Source: CAD feature listing. Evaluate the final solid. Frame: model axes, mm. Face numbers are marked on the shaded views. A direction names the side the tool comes from. Give positions to 0.01 mm unless a question says otherwise; leave off trailing zeros.
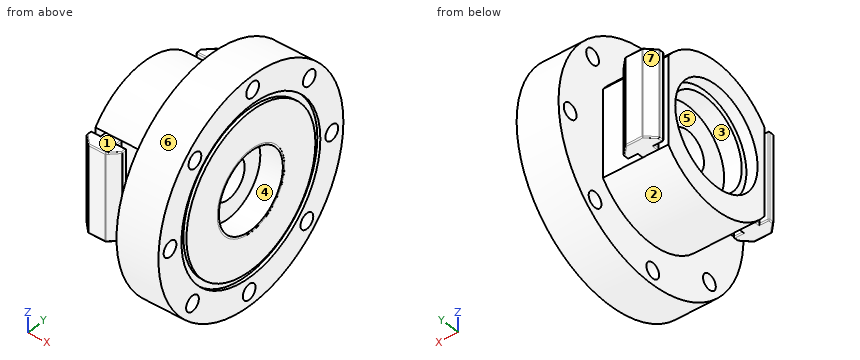
```python
from build123d import *

# Parameters (mm, degrees)
M6_CLEARANCE_HOLE1_D = 7
SKETCH4_W            = 29.717000002
SKETCH4_H            = 66.04
CUT_EXTRUDE1_DEPTH   = 6.5786
BOSS_EXTRUDE1_DEPTH  = 39.556176
FILLET1_R            = 0.508
FILLET1_OF_MIRROR1_R = 0.508


with BuildPart() as part:
    # Main sketch → Revolve1 (revolve)
    with BuildSketch(Plane.XY):
        Polygon((0, 9.000000034), (0, 20.074999982), (-8.000000002, 20.074999982), (-8.000000002, 22.614999982), (-13.080000002, 22.614999982), (-13.080000002, 33.02), (-8.000000002, 33.02), (16.637, 33.02), (16.637, 50.8), (35.687, 50.8), (35.687, 38.1508), (34.3154, 38.1508), (34.3154, 35.433), (35.687, 35.433), (35.687, 18.4912), (35.6616, 18.4912), (35.6616, 17.6022), (25.4, 17.6022), (25.4, 9.000000034), align=None)
    revolve(axis=Axis((71.950113838, 0, 0), (-1, 0, 0)))

    # M6 Clearance Hole1 (through all)
    with Locations(Plane(origin=(35.687, 0, 0), x_dir=(0, 0, -1), z_dir=(1, 0, 0))):
        with Locations((0, 0), (-44.439876155, 0.948634466), (-32.094523648, -30.75295192), (-0.948634466, -44.439876155), (30.75295192, -32.094523648), (44.439876155, -0.948634466), (32.094523648, 30.75295192), (0.948634466, 44.439876155), (-30.75295192, 32.094523648)):
            Hole(M6_CLEARANCE_HOLE1_D / 2)

    # Sketch4 → Cut-Extrude1 (cut)
    with BuildSketch(Plane(origin=(0, 33.02, 0), x_dir=(1, 0, 0), z_dir=(0, 1, 0))):
        with Locations((1.778499999, 0)):
            Rectangle(SKETCH4_W, SKETCH4_H)
    cut_extrude1 = extrude(amount=-CUT_EXTRUDE1_DEPTH, mode=Mode.SUBTRACT)

    # Sketch5 → Boss-Extrude1 (add)
    with BuildSketch(Plane(origin=(0, 0, 19.778088028), x_dir=(-1, 0, 0), z_dir=(0, 0, -1))):
        Polygon((1.191199802, 26.4414), (1.191199802, 28.868399972), (-3.175999998, 28.868399972), (-3.175999998, 31.327400134), (0.988799902, 35.492200034), (8.915200102, 35.492200034), (13.080000002, 31.327400134), (13.080000002, 28.868399972), (8.712800202, 28.868399972), (8.712800202, 26.4414), align=None)
    boss_extrude1 = extrude(amount=BOSS_EXTRUDE1_DEPTH)

    # Fillet1
    fillet1_edges = [part.edges().sort_by_distance(p)[0] for p in [
        (-8.712800202, 27.654899986, -19.778087972),
        (-8.712800202, 27.654899986, 19.778088028),
        (-10.896400102, 28.868399972, -19.778087972),
        (-10.896400102, 28.868399972, 19.778088028),
        (-13.080000002, 30.097900053, -19.778087972),
        (-13.080000002, 28.868399972, 2.8e-08),
        (-13.080000002, 30.097900053, 19.778088028),
        (-10.997600052, 33.409800084, -19.778087972),
        (-13.080000002, 31.327400134, 2.8e-08),
        (-10.997600052, 33.409800084, 19.778088028),
        (-8.915200102, 35.492200034, 2.8e-08),
        (-0.988799902, 35.492200034, 2.8e-08),
        (3.175999998, 31.327400134, 2.8e-08),
        (3.175999998, 28.868399972, 2.8e-08),
        (-1.191199802, 27.654899986, 19.778088028),
        (0.992400098, 28.868399972, 19.778088028),
        (3.175999998, 30.097900053, 19.778088028),
        (1.093600048, 33.409800084, 19.778088028),
        (-4.952000002, 35.492200034, 19.778088028),
        (-4.952000002, 35.492200034, -19.778087972),
        (1.093600048, 33.409800084, -19.778087972),
        (3.175999998, 30.097900053, -19.778087972),
        (0.992400098, 28.868399972, -19.778087972),
        (-1.191199802, 27.654899986, -19.778087972),
    ]]
    fillet(fillet1_edges, radius=FILLET1_R)

    # Mirror1: Cut-Extrude1, Boss-Extrude1 across plane
    add(cut_extrude1.mirror(Plane.ZX), mode=Mode.SUBTRACT)
    add(boss_extrude1.mirror(Plane.ZX))

    # Fillet1 of Mirror1
    fillet1_of_mirror1_edges = [part.edges().sort_by_distance(p)[0] for p in [
        (-8.712800202, -27.654899986, -19.778087972),
        (-8.712800202, -27.654899986, 19.778088028),
        (-10.896400102, -28.868399972, -19.778087972),
        (-10.896400102, -28.868399972, 19.778088028),
        (-13.080000002, -30.097900053, -19.778087972),
        (-13.080000002, -28.868399972, 2.8e-08),
        (-13.080000002, -30.097900053, 19.778088028),
        (-10.997600052, -33.409800084, -19.778087972),
        (-13.080000002, -31.327400134, 2.8e-08),
        (-10.997600052, -33.409800084, 19.778088028),
        (-8.915200102, -35.492200034, 2.8e-08),
        (-0.988799902, -35.492200034, 2.8e-08),
        (3.175999998, -31.327400134, 2.8e-08),
        (3.175999998, -28.868399972, 2.8e-08),
        (-1.191199802, -27.654899986, 19.778088028),
        (0.992400098, -28.868399972, 19.778088028),
        (3.175999998, -30.097900053, 19.778088028),
        (1.093600048, -33.409800084, 19.778088028),
        (-4.952000002, -35.492200034, 19.778088028),
        (-4.952000002, -35.492200034, -19.778087972),
        (1.093600048, -33.409800084, -19.778087972),
        (3.175999998, -30.097900053, -19.778087972),
        (0.992400098, -28.868399972, -19.778087972),
        (-1.191199802, -27.654899986, -19.778087972),
    ]]
    fillet(fillet1_of_mirror1_edges, radius=FILLET1_OF_MIRROR1_R)


solid = part.part
```
1) Material intervals for L1, parallel to Y at x = -9.4, z = 0 (3 decimals); L2, parallel to Y at x = -4, z = 0 (3 decimals); L3, parallel to Z at x = 23, y = 29.5, sorted ascending.
Report:
L1: y = -35.007 to -28.868, -26.441 to -22.615, 22.615 to 26.441, 28.868 to 35.007
L2: y = -35.492 to -20.075, 20.075 to 35.492
L3: z = -41.36 to -35.36, -28.83 to 28.4, 33.1 to 41.36
2) Reachability of the marked faces 1, 2, 3 and 4 from +Z, -Z, +X, -X, +Y, -Y: full face, straight path, thin tool, end or side. Return the list, or none.
Report:
face 1: +Z, -X, -Y
face 2: -Z, -X
face 3: -X
face 4: +X
3) Draft query along Y for the marked faces 5, 6 and 7. Return one class per face: +Y half, -Y half, draft (parallel to the pull), parting line (faces both ways), or undercut.
Report:
face 5: undercut
face 6: parting line
face 7: +Y half
4) Section query A-A, the plane x = 27. Count the separate pieces of the cut face and the enclosed holes in it, and give its area (3 significant figures).
Report:
separate pieces: 1
enclosed holes: 9
area: 6,830 mm2
5) Pin query (flat end, axial travel): pin 1 (3 mm diameter, centred on x = 0.5, z = 36, fed in from +Y); pin 2 (9.5 mm diameter, centred on x = -8.5, y = -30.5, fed in from -Z); pin 3 (5.5 mm diameter, centred on x = 9, z = 1.5, fed in from -Y); pin 4 (0.7 mm diameter, centred on y = -27.5, z = 3.5, fed in from -X). Return the tip coordinate at first contact, or that it passes through.
Report:
pin 1: passes through
pin 2: stops at z = -20.67
pin 3: stops at y = -26.44
pin 4: stops at x = -8.71
